Could you check a few things on this drawing? It's one solid part, dimensions in mm from its lowest x, y, z. A direction names the side the tool comes from. Give positions to 0.01 mm unless a question says otherwise; leave off trailing zeros. Loops run counter-clockwise (first coordinate to the right, second up) from the corner with the lowest first, then second, coordinate; pieces in that order, holes last. Notation, with made-up numbers: (-19.5, 34.5) - (30.5, 34.5) arc R15 ccw to (30.5, 57.5) - close; hole circle Ø1 at (29.5, 61.25). An arc over 180 degrees is marked (long way). Return JSON: item names as keys, results as strings. Group by question number.
(1) If we section it at A-A (z = 200): Please give me the cut outline in (x, y), then the cut area to 3 significant figures.
(2) If we section it at C-C (x = 222): Please give me the cut outline in (y, z).
(3) For P1, Ø1.5, axis at x = 352.5, y = 318, coming from the -Z side; P2, Ø18, axis at x = 50, y = 200, coming from the -Z side; P3, Ø5, axis at x = 132, z = 354, coming from the -Y side, each with a flat end and sliding along its axis, tell me the tip position at first contact or that it passes through.
(4) If we section it at D-D (x = 79): Please give me the cut outline in (y, z), then the cut area to 3 significant figures.
(5) I need wall thicknesses on probe 1 along Y at (x, z) = (290, 200); probe 2 along X at (y, z) = (200, 245); probe 3 along Z at (x, y) = (97, 200). Which ranges of each line are inside material? Lowest first, please. Write a range as [from, to].
(6) If we section it at B-B (y = 200): Please give me the cut outline in (x, z).
(7) On a 3-axis mill with a long thin cutter (end or side, diameter ignored), from which of +Z, -Z, +X, -X, +Y, -Y can I reach the whole of each face in a straight line? I mean the marked faces 1 and 2. Say none if no direction works.
(8) If we mould it in two halves opening along Z, with no side actions, what happens to the marked faces 3, 4 and 5? For each: released by +Z, released by -Z, zero draft, split by the parting line, or undercut.
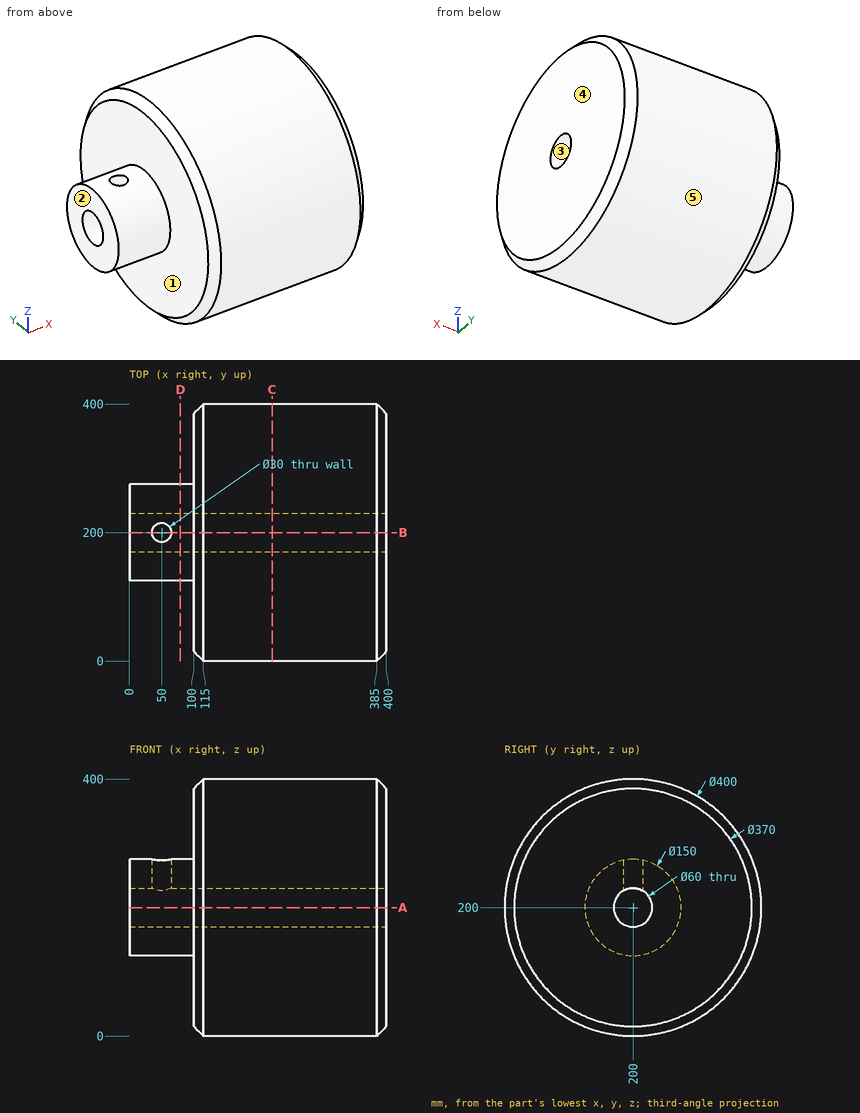
Values:
{
 "1": {"outline": "(0, 125) - (100, 125) - (100, 15) - (115, 0) - (385, 0) - (400, 15) - (400, 170) - (0, 170) - close; (0, 230) - (400, 230) - (400, 385) - (385, 400) - (115, 400) - (100, 385) - (100, 275) - (0, 275) - close", "area": "111,000 mm2"},
 "2": {"outline": "circle Ø400 at (200, 200); hole circle Ø60 at (200, 200)"},
 "3": {"P1": "z = 37.97", "P2": "z = 125", "P3": "y = 69.43"},
 "4": {"outline": "circle Ø150 at (200, 200); hole circle Ø60 at (200, 200)", "area": "14,800 mm2"},
 "5": {"probe 1": "[0, 170], [230, 400]", "probe 2": "[0, 35], [65, 400]", "probe 3": "[125, 170], [230, 275]"},
 "6": {"outline": "(0, 125) - (100, 125) - (100, 15) - (115, 0) - (385, 0) - (400, 15) - (400, 170) - (0, 170) - close; (0, 230) - (35, 230) - (35, 275) - (0, 275) - close; (65, 230) - (400, 230) - (400, 385) - (385, 400) - (115, 400) - (100, 385) - (100, 275) - (65, 275) - close"},
 "7": {"face 1": "-X", "face 2": "+Z, -Z, -X, +Y, -Y"},
 "8": {"face 3": "undercut", "face 4": "zero draft", "face 5": "split by the parting line"}
}
